from build123d import *

# Parameters (mm, degrees)
F1_DEPTH = 25.4
F2_T     = -1.5875
F3_W     = 22.225
F3_H     = 22.225
F4_DEPTH = 262.563512
F6_DEPTH = 25.4


with BuildPart() as f1:
    # F0 (on Top) → F1 (new body)
    with BuildSketch(Plane.XY):
        Polygon((5.260512, 127.561512), (-12.7, 109.601), (-12.7, -135.001), (12.7, -135.001), (12.7, 120.122024), align=None)
    extrude(amount=F1_DEPTH)

    # F2
    f2_openings = [f1.faces().sort_by_distance(p)[0] for p in [
        (0, -135.001, 12.7),
    ]]
    offset(amount=F2_T, openings=f2_openings)

    # F3 (on face) → F4 (cut, through all)
    with BuildSketch(Plane.XZ.offset(135.001)):
        with Locations((0, 12.7)):
            Rectangle(F3_W, F3_H)
    extrude(amount=-F4_DEPTH, mode=Mode.SUBTRACT)

    # F5 (on face) → F6 (cut)
    with BuildSketch(Plane.XY.offset(25.4)):
        Polygon((12.7, -109.601), (-12.7, -135.001), (12.7, -135.001), align=None)
    extrude(amount=-F6_DEPTH, mode=Mode.SUBTRACT)


solid = f1.part
Model file for the job. Use its own axes, mm. A direction names the side the tool comes from. Give positions to 0.01 mm unless a question says otherwise; leave off trailing zeros. Loops run counter-clockwise (first coordinate to the right, second up) from the corner with the lowest first, then second, coordinate; pieces in that order, holes last.
1) Pull direction Z, two halves, no side cores. Call faces 3 (the flat face through (11.48, 121.34, 12.64)), 4 (the flat face through (0, -2, 25.4)), 5 (the flat face through (0, -1, 1.588)), 6 (the flat face through (0, -2, 0)): +Z half, -Z half, draft (parallel to the pull), parting line (faces both ways), or undercut.
2) Saw through at A-A (z = 13.5). Write the cut outline in (x, y), plus the area to 3 significant figures.
3) Flat gauge pin, fed straight in: pin 1 Ø11 at (x, y) = (-1, 26) entering from -Z. Where does the tip first touch, or does it go through?
4) Wall check: line 1 (Z direction, x = 3, y = -8); line 2 (X direction, y = 47, z = 13.5); line 3 (Y direction, x = 11.5, z = 5). Give the ranges that are in metal, low to high.
5) Saw through at B-B (y = -13). Write the cut outline in (x, z).
6) Saw through at C-C (x = 2.25). Write the cut outline in (y, z).
7) Tool access for faces 1 (the flat face through (0.1, -122.2, 24)), 2 (the flat face through (0, -1, 23.812)): list every direction of +Z, -Z, +X, -X, +Y, -Y with a clear straight run to the whole face (end or side of a thin tool).
Answer block:
1. face 3: draft
1. face 4: +Z half
1. face 5: undercut
1. face 6: -Z half
2. outline: (-12.7, -135) - (-11.11, -133.41) - (-11.11, 111.19) - (-12.7, 109.6) - close; (11.11, -111.19) - (12.7, -109.6) - (12.7, 120.12) - (11.11, 121.71) - close
2. area: 756 mm2
3. pin 1: stops at z = 0
4. line 1: z = 0 to 1.59, 23.81 to 25.4
4. line 2: x = -12.7 to -11.11, 11.11 to 12.7
4. line 3: y = -110.8 to 121.32
5. outline: (-12.7, 0) - (12.7, 0) - (12.7, 25.4) - (-12.7, 25.4) - close; hole (-11.11, 1.59) - (11.11, 1.59) - (11.11, 23.81) - (-11.11, 23.81) - close
6. outline: (-120.05, 0) - (124.55, 0) - (124.55, 1.59) - (-120.05, 1.59) - close; (-120.05, 23.81) - (124.55, 23.81) - (124.55, 25.4) - (-120.05, 25.4) - close
7. face 1: +Z, -Z, +X, -Y
7. face 2: +Y, -Y
